```python
from build123d import *

# Parameters (mm, degrees)
BOSS_EXTRUDE1_DEPTH           = 22.5
BOSS_EXTRUDE1_DEPTH_BACK      = 22.5
SKETCH8_W                     = 10
SKETCH8_H                     = 120
BOSS_EXTRUDE2_DEPTH           = 30
M8_CLEARANCE_HOLE2_AT_2_COUNT = 2
M8_CLEARANCE_HOLE2_AT_2_PITCH = 90.58835466
M8_CLEARANCE_HOLE2_AT_3_COUNT = 2
M8_CLEARANCE_HOLE2_AT_3_PITCH = 42.5
BOSS_EXTRUDE3_REACH           = 134.793
SKETCH2_R                     = 2.38
CUT_EXTRUDE1_DEPTH            = 60
CHAMFER4_SIZE                 = 10
CHAMFER4_SIZE_2               = 12.433047379
SKETCH18_R                    = 7.5
CUT_EXTRUDE4_DEPTH            = 85
SKETCH19_W                    = 61.758143573
SKETCH19_H                    = 25.520807093
CUT_EXTRUDE5_DEPTH            = 10


with BuildPart() as part:
    # Sketch1 → Boss-Extrude1 (new, two sides: drawn at the far end of the back side and taken through both)
    with BuildSketch(Plane.XY.offset(-BOSS_EXTRUDE1_DEPTH_BACK)):
        Polygon((0, 60), (10, 60), (10, -21.4124), (91.7, -21.4124), (91.7, -31.4124), (10, -31.4124), (10, -60), (0, -60), align=None)
    extrude(amount=BOSS_EXTRUDE1_DEPTH + BOSS_EXTRUDE1_DEPTH_BACK)

    # Sketch8 → Boss-Extrude2 (add)
    with BuildSketch(Plane(origin=(0, 0, -22.5), x_dir=(-1, 0, 0), z_dir=(0, 0, -1))):
        with Locations((-5, 0)):
            Rectangle(SKETCH8_W, SKETCH8_H)
    boss_extrude2 = extrude(amount=BOSS_EXTRUDE2_DEPTH)

    # Sketch10 → M8 Clearance Hole2 (revolve, cut)
    with BuildSketch(Plane(origin=(10, 40, 0), x_dir=(0, 0, -1), z_dir=(0, 1, 0))):
        Polygon((0, 0), (0, 25.703872786), (4.5, 23), (4.5, 0.025), (4.525, 0), align=None)
    m8_clearance_hole2 = revolve(axis=Axis((16.35, 40, 0), (-1, 0, 0)), mode=Mode.SUBTRACT)

    # M8 Clearance Hole2 at 2: M8 Clearance Hole2 ×2
    with Locations(*[Vector(0, -0.8831157194574106, -0.4691552259617494) * (i * M8_CLEARANCE_HOLE2_AT_2_PITCH) for i in range(1, M8_CLEARANCE_HOLE2_AT_2_COUNT)]):
        add(m8_clearance_hole2, mode=Mode.SUBTRACT)

    # M8 Clearance Hole2 at 3: M8 Clearance Hole2 ×2
    with Locations(*[(0, 0, -i * M8_CLEARANCE_HOLE2_AT_3_PITCH) for i in range(1, M8_CLEARANCE_HOLE2_AT_3_COUNT)]):
        add(m8_clearance_hole2, mode=Mode.SUBTRACT)

    # Boss-Extrude3: up to this face of the body (flat: up to its plane)
    boss_extrude3_end = Plane(part.part.faces().sort_by_distance((50.85, -26.4124, -22.5))[0])
    # Sketch14 → Boss-Extrude3 (add, up to the picked face)
    with BuildSketch(Plane.XY.offset(22.5), mode=Mode.PRIVATE) as boss_extrude3_sk1:
        Polygon((91.7, -21.4124), (10, 38.5), (10, -21.4124), align=None)
    boss_extrude3_tool1 = split(extrude(boss_extrude3_sk1.sketch, amount=-BOSS_EXTRUDE3_REACH, mode=Mode.PRIVATE), bisect_by=boss_extrude3_end, keep=Keep.BOTH, mode=Mode.PRIVATE)
    add(boss_extrude3_tool1.solids().sort_by(Axis((37.233333, -1.4416, 22.5), (0, 0, -1)))[0])

    # Sketch2 → Cut-Extrude1 (cut)
    with BuildSketch(Plane(origin=(0, -31.4124, 0), x_dir=(1, 0, 0), z_dir=(0, 1, 0))):
        with Locations((68.7, 10.325)):
            Circle(SKETCH2_R)
        with Locations((68.7, -10.325)):
            Circle(SKETCH2_R)
        with Locations((29, 10.325)):
            Circle(SKETCH2_R)
        with Locations((29, -10.325)):
            Circle(SKETCH2_R)
    extrude(amount=CUT_EXTRUDE1_DEPTH, mode=Mode.SUBTRACT)

    # Mirror2: Boss-Extrude2, M8 Clearance Hole2 across plane
    add(boss_extrude2.mirror(Plane.XY))
    add(m8_clearance_hole2.mirror(Plane.XY), mode=Mode.SUBTRACT)

    # Mirror2 copy 1 sketch → Mirror2 copy 1 (revolve, cut)
    with BuildSketch(Plane(origin=(10, -40, 42.5), x_dir=(0, 0, 1), z_dir=(0, 1, 0))):
        Polygon((0, 0), (0, -25.703872786), (4.5, -23), (4.5, -0.025), (4.525, 0), align=None)
    revolve(axis=Axis((16.35, -40, 42.5), (1, 0, 0)), mode=Mode.SUBTRACT)

    # Mirror2 copy 2 sketch → Mirror2 copy 2 (revolve, cut)
    with BuildSketch(Plane(origin=(10, 40, 42.5), x_dir=(0, 0, 1), z_dir=(0, 1, 0))):
        Polygon((0, 0), (0, -25.703872786), (4.5, -23), (4.5, -0.025), (4.525, 0), align=None)
    revolve(axis=Axis((16.35, 40, 42.5), (1, 0, 0)), mode=Mode.SUBTRACT)

    # Chamfer4
    # the kernel refuses this chamfer: 12.433047379, 10 mm, written as the material it takes off along each edge
    with BuildSketch(Plane(origin=(10, -60, 84.560907877), x_dir=(0.03755485384602002, 0.9992945676589081, 0), z_dir=(0, 0, -1))) as chamfer4_piece_1:
        Polygon((CHAMFER4_SIZE * 0.999294567659, -CHAMFER4_SIZE * 0.037554853846), (-CHAMFER4_SIZE_2 * 0.037554853846, -CHAMFER4_SIZE_2 * 0.999294567658), (0, 0), align=None)
    extrude(amount=169.121815753, mode=Mode.SUBTRACT)

    # Sketch18 → Cut-Extrude4 (cut)
    with BuildSketch(Plane(origin=(0, 60, 0), x_dir=(1, 0, 0), z_dir=(0, 1, 0))):
        with Locations(Location((29, 10.325, 0), (0, 0, 270))):
            Circle(SKETCH18_R)
        with Locations(Location((29, -10.325, 0), (0, 0, 270))):
            Circle(SKETCH18_R)
        with Locations(Location((68.7, 10.325, 0), (0, 0, 270))):
            Circle(SKETCH18_R)
        with Locations(Location((68.7, -10.325, 0), (0, 0, 270))):
            Circle(SKETCH18_R)
    extrude(amount=-CUT_EXTRUDE4_DEPTH, mode=Mode.SUBTRACT)

    # Sketch19 → Cut-Extrude5 (cut)
    with BuildSketch(Plane(origin=(91.7, 0, 0), x_dir=(0, 0, -1), z_dir=(1, 0, 0))):
        with Locations((3.038191321, -4.992790305)):
            Rectangle(SKETCH19_W, SKETCH19_H)
    extrude(amount=-CUT_EXTRUDE5_DEPTH, mode=Mode.SUBTRACT)


solid = part.part
```
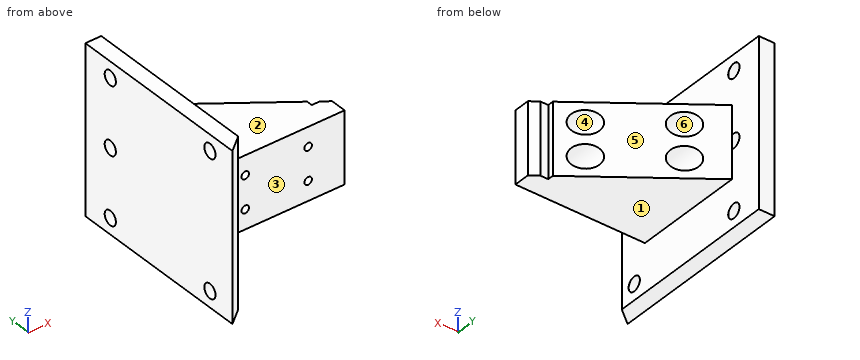
Geometry check sheet. Reference: the model listing, model coordinates, mm. Face numbers are marked on the shaded views. A direction names the side the tool comes from. Give positions to 0.01 mm unless a question says otherwise; leave off trailing zeros. Order: outer loops, then holes, each group sorted by start corner. A loop starts at its lowest first (then second) coordinate and runs counter-clockwise, first axis right, second up. Notation, with made-up numbers: (37.5, 12.5) - (66.5, 12.5) arc R15 cw to (66.5, 33.5) - close; hole circle Ø6 at (69, -28). An arc over 180 degrees is marked (long way). Answer in a Markdown table with one row per item. Add a question column.
Q1. Gauge pin test, flat ends, axial feed: pin 1 (8 mm diameter, centred on x = 40, z = -15.5, fed in from -Y); pin 2 (2 mm diameter, centred on x = 16.5, z = -11.5, fed in from +Y); pin 3 (4 mm diameter, centred on x = 68.7, z = 10.325, fed in from +Y); pin 4 (5.5 mm diameter, centred on x = 84, z = 5, fed in from +Y). Record the tip position at first contact, or that the pin passes through.
Q2. Mould release check, pull along Z, two halves, no side actions. Record for the marked faces 1, 2, 3 and 4: pulls with the +Z half, pulls with the -Z half, needs draft (parallel to the pull), parting line crosses it, or undercut.
Q3. Tool access check on the marked faces 5 and 6. Record the directions out of +Z, -Z, +X, -X, +Y, -Y that give a thin tool (end or side, any length) a straight path to the whole face; none if there is none.
Q4. Material ranges on probe 1 along Z at (x, y) = (7.25, -40); probe 2 along Z at (x, y) = (68.7, -29.5) (3 decimals); probe 3 along Y at (x, z) = (4.25, -42.5), recorded low to high. Write a range as from..to.
Q5. Cross-section at A-A, the plane z = -42.5. Enter the section's corners in (x, y) (3 decimals), then the cut area to 3 significant figures.
Q6. Cross-section at B-B, the plane y = 40. Enter the section's corners in (x, z) (3 decimals).
Q7. Cross-section at D-D, the plane x = 68.7. Enter the section's corners in (y, z) (3 decimals), then the cut area to 3 significant figures.
Q8. Cross-section at C-C, the plane z = 0. Enter the section's corners in (x, y) (3 decimals), then the cut area to 3 significant figures.
Check values:
| question | item | result |
|---|---|---|
| 1 | pin 1 | stops at y = -31.41 |
| 1 | pin 2 | stops at y = 34.47 |
| 1 | pin 3 | passes through |
| 1 | pin 4 | stops at y = -13.75 |
| 2 | face 1 | pulls with the -Z half |
| 2 | face 2 | pulls with the +Z half |
| 2 | face 3 | needs draft |
| 2 | face 4 | undercut |
| 3 | face 5 | +Z, -Z, +X, +Y |
| 3 | face 6 | +Y |
| 4 | probe 1 | z = -52.5..-47, -38..38, 47..52.5 |
| 4 | probe 2 | z = -22.5..-12.705, -7.945..7.945, 12.705..22.5 |
| 4 | probe 3 | y = -54.62..-44.5, -35.5..35.5, 44.5..60 |
| 5 | outline | (0, -58.043) - (10, -50) - (10, -44.525) - (9.975, -44.5) - (0, -44.5) - close; (0, -35.5) - (9.975, -35.5) - (10, -35.475) - (10, 35.475) - (9.975, 35.5) - (0, 35.5) - close; (0, 44.5) - (9.975, 44.5) - (10, 44.525) - (10, 60) - (0, 60) - close |
| 5 | area | 960 mm^2 |
| 6 | outline | (0, -52.5) - (10, -52.5) - (10, -47.025) - (9.975, -47) - (0, -47) - close; (0, -38) - (9.975, -38) - (10, -37.975) - (10, -4.525) - (9.975, -4.5) - (0, -4.5) - close; (0, 4.5) - (9.975, 4.5) - (10, 4.525) - (10, 37.975) - (9.975, 38) - (0, 38) - close; (0, 47) - (9.975, 47) - (10, 47.025) - (10, 52.5) - (0, 52.5) - close |
| 7 | outline | (-31.412, -22.5) - (-4.546, -22.5) - (-4.546, -17.825) - (-25, -17.825) - (-25, -12.705) - (-31.412, -12.705) - close; (-31.412, -7.945) - (-25, -7.945) - (-25, -2.825) - (-4.546, -2.825) - (-4.546, 2.825) - (-25, 2.825) - (-25, 7.945) - (-31.412, 7.945) - close; (-31.412, 12.705) - (-25, 12.705) - (-25, 17.825) - (-4.546, 17.825) - (-4.546, 22.5) - (-31.412, 22.5) - close |
| 7 | area | 534 mm^2 |
| 8 | outline | (0, -58.043) - (10, -50) - (10, -31.412) - (91.7, -31.412) - (91.7, -21.412) - (86.71, -17.753) - (81.7, -17.753) - (81.7, -14.079) - (10, 38.5) - (10, 35.475) - (9.975, 35.5) - (0, 35.5) - close; (0, 44.5) - (9.975, 44.5) - (10, 44.525) - (10, 60) - (0, 60) - close |
| 8 | area | 4,310 mm^2 |
